```python
from build123d import *

# Parameters (mm, degrees)
SKETCH1_W               = 711.2
SKETCH1_H               = 685.8
BOSS_EXTRUDE1_DEPTH     = 3.175
SKETCH2_W               = 635
SKETCH2_H               = 666.75
BOSS_EXTRUDE2_DEPTH     = 50.8
CUT_EXTRUDE1_DEPTH      = 497.935680571
CUT_EXTRUDE1_DEPTH_BACK = 497.935680571
SKETCH4_W               = 19.05
SKETCH4_H               = 666.75
BOSS_EXTRUDE3_DEPTH     = 3.175
SKETCH5_W               = 317.5
SKETCH5_H               = 6.35
CUT_EXTRUDE2_DEPTH      = 19.05
FILLET1_R               = 43.18
SKETCH6_W               = 635
SKETCH6_H               = 152.4
BOSS_EXTRUDE4_DEPTH     = 15.24
DRAFT2_ANGLE            = 11
SHELL1_START            = -314.325
SHELL1_DEPTH            = 628.65
SHELL1_START_2          = -333.375
SHELL1_2_OUTLINE_W      = 3.175
SHELL1_2_OUTLINE_H      = 663.575
SHELL1_2_DEPTH          = 666.75
SKETCH7_W               = 127
SKETCH7_H               = 127
CUT_EXTRUDE3_DEPTH      = 25.4
LPATTERN1_COUNT         = 4
LPATTERN1_PITCH         = 160.02
FILLET2_R               = 12.7


# Read off the part's stored shape, not the designer's step: Shell1
with BuildPart() as part:
    # Sketch1 → Boss-Extrude1 (new body)
    with BuildSketch(Plane(origin=(0, 0, 0), x_dir=(1, 0, 0), z_dir=(0, 1, 0))):
        Rectangle(SKETCH1_W, SKETCH1_H)
    extrude(amount=BOSS_EXTRUDE1_DEPTH)

    # Sketch2 → Boss-Extrude2 (add)
    with BuildSketch(Plane(origin=(0, 3.175, 0), x_dir=(1, 0, 0), z_dir=(0, 1, 0))):
        with Locations((0, 9.525)):
            Rectangle(SKETCH2_W, SKETCH2_H)
    extrude(amount=BOSS_EXTRUDE2_DEPTH)

    # Sketch3 → Cut-Extrude1 (cut, two sides: drawn at the far end of the back side and taken through both)
    with BuildSketch(Plane(origin=(0, 0, 0), x_dir=(0, 0, -1), z_dir=(1, 0, 0)).offset(-CUT_EXTRUDE1_DEPTH_BACK)):
        Polygon((-196.85, 53.975), (-170.68027758, 44.45), (342.9, 44.45), (342.9, 53.975), align=None)
    extrude(amount=CUT_EXTRUDE1_DEPTH + CUT_EXTRUDE1_DEPTH_BACK, mode=Mode.SUBTRACT)

    # Sketch4 → Boss-Extrude3 (add)
    with BuildSketch(Plane(origin=(0, 3.175, 0), x_dir=(1, 0, 0), z_dir=(0, 1, 0))):
        with Locations((-327.025, 9.525)):
            Rectangle(SKETCH4_W, SKETCH4_H)
    boss_extrude3 = extrude(amount=BOSS_EXTRUDE3_DEPTH)

    # Mirror1: Boss-Extrude3 across plane
    add(boss_extrude3.mirror(Plane(origin=(0, 0, 0), x_dir=(0, 0, 1), z_dir=(1, 0, 0))))

    # Sketch5 → Cut-Extrude2 (cut)
    with BuildSketch(Plane(origin=(0, 0, -342.9), x_dir=(-1, 0, 0), z_dir=(0, 0, -1))):
        with Locations((-158.75, 41.275)):
            Rectangle(SKETCH5_W, SKETCH5_H)
    cut_extrude2 = extrude(amount=-CUT_EXTRUDE2_DEPTH, mode=Mode.SUBTRACT)

    # Mirror2: Cut-Extrude2 across plane
    add(cut_extrude2.mirror(Plane(origin=(0, 0, 0), x_dir=(0, 0, 1), z_dir=(1, 0, 0))), mode=Mode.SUBTRACT)

    # Fillet1
    fillet1_edges = [part.edges().sort_by_distance(p)[0] for p in [
        (0, 53.975, 323.85),
    ]]
    fillet(fillet1_edges, radius=FILLET1_R)

    # Sketch6 → Boss-Extrude4 (add)
    with BuildSketch(Plane(origin=(0, 44.45, 0), x_dir=(1, 0, 0), z_dir=(0, 1, 0))):
        with Locations((0, 222.25)):
            Rectangle(SKETCH6_W, SKETCH6_H)
    extrude(amount=BOSS_EXTRUDE4_DEPTH)

    # Draft2
    draft2_faces = [part.faces().sort_by_distance(p)[0] for p in [
        (0, 52.07, -146.05),
        (0, 52.07, -298.45),
    ]]
    draft(draft2_faces, Plane.ZX.offset(59.69), DRAFT2_ANGLE)

    # Shell1 outline → Shell1 (cut)
    with BuildSketch(Plane.YZ.offset(SHELL1_START)):
        with BuildLine():
            Line((41.275, -145.704912114), (41.275, 171.240115743))
            Line((41.275, 171.240115743), (50.8, 197.409838164))
            Line((50.8, 197.409838164), (50.8, 280.67))
            ThreePointArc((50.8, 280.67), (39.082806781, 308.957806781), (10.795, 320.675))
            Line((10.795, 320.675), (0, 320.675))
            Line((0, 320.675), (0, -342.9))
            Line((0, -342.9), (34.925, -342.9))
            Line((34.925, -342.9), (34.925, -320.675))
            Line((34.925, -320.675), (41.275, -320.675))
            Line((41.275, -320.675), (41.275, -298.795087886))
            Line((41.275, -298.795087886), (56.515, -295.832731975))
            Line((56.515, -295.832731975), (56.515, -148.667268025))
            Line((56.515, -148.667268025), (41.275, -145.704912114))
        make_face()
    extrude(amount=SHELL1_DEPTH, mode=Mode.SUBTRACT)

    # Shell1 2 outline → Shell1 2 (cut)
    with BuildSketch(Plane.YZ.offset(SHELL1_START_2)):
        with Locations((1.5875, -11.1125)):
            Rectangle(SHELL1_2_OUTLINE_W, SHELL1_2_OUTLINE_H)
    extrude(amount=SHELL1_2_DEPTH, mode=Mode.SUBTRACT)

    # Sketch7 → Cut-Extrude3 (cut)
    with BuildSketch(Plane(origin=(0, 59.69, 0), x_dir=(1, 0, 0), z_dir=(0, 1, 0))):
        with Locations((-241.3, 222.25)):
            Rectangle(SKETCH7_W, SKETCH7_H)
    cut_extrude3 = extrude(amount=-CUT_EXTRUDE3_DEPTH, mode=Mode.SUBTRACT)

    # LPattern1: Cut-Extrude3 ×4
    with Locations(*[(i * LPATTERN1_PITCH, 0, 0) for i in range(1, LPATTERN1_COUNT)]):
        add(cut_extrude3, mode=Mode.SUBTRACT)

    # Fillet2
    fillet2_edges = [part.edges().sort_by_distance(p)[0] for p in [
        (-304.8, 58.1025, -158.75),
        (-304.8, 58.1025, -285.75),
        (-177.8, 58.1025, -285.75),
        (-177.8, 58.1025, -158.75),
    ]]
    fillet(fillet2_edges, radius=FILLET2_R)


solid = part.part
```
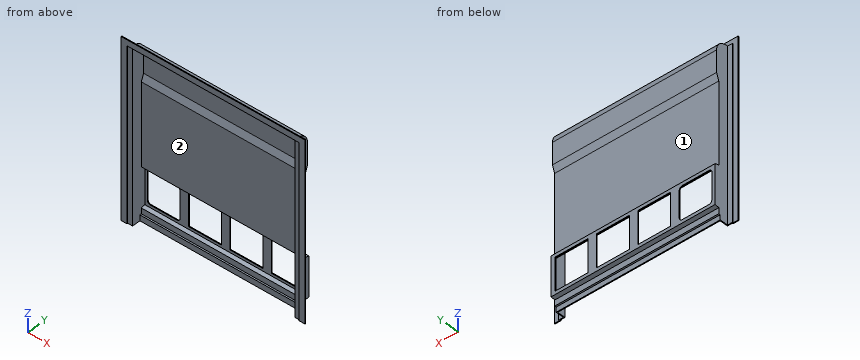
Input: part model. Units: mm. Frame: model coordinates. Face numbers are marked on the shaded views. Give positions to 0.01 mm unless a question says otherwise; leave off trailing zeros. Write each loop counter-clockwise with the first axis right and the second up, starting at its lowest first coordinate (ties: lowest second). Pieces come first, ordered by that corner, then holes. Notation, with made-up numbers: (-19.5, 54.5) - (8.5, 54.5) arc R24 ccw to (8.5, 65.5) - close; hole circle Ø1 at (65.25, 39.5). An arc over 180 degrees is marked (long way). Write item = value, one per line. Start each with the question number.
1) Material intervals for L1, parallel to Z at x = -94, y = 57; L2, parallel to X at y = 40, z = -42.5 (3 decimals); L3, parallel to X at y = 3.5, z = -285 (3 decimals), sorted ascending. Write a range as [from, to].
2) Cut plane B-B (z = 5). Return loops of the section in (x, y) (3 decimals).
3) Draft query along X for the marked faces 1 and 2. Return one class per face: pulls with the +X half, pulls with the -X half, needs draft (parallel to the pull), parting line crosses it, or undercut.
4) Cut plane C-C (x = 156). Return loops of the section in (y, z) (3 decimals), and give its area (3 significant figures).
5) Pin query (flat end, axial travel): pin 1 (4 mm diameter, centred on x = -123, y = 8.5, fed in from +Z); pin 2 (1.6 mm diameter, centred on y = 58, z = -228, fed in from -X); pin 3 (8 mm diameter, centred on y = 18.5, z = 196, fed in from +X). Return the tip coordinate at first contact, or that it passes through.
6) Cut plane D-D (y = 20.5). Return loops of the section in (x, z) (3 decimals).
Answers follow:
q1.L1 = [-298.97, -285.75], [-158.75, -145.53]
q1.L2 = [-317.5, -314.325], [314.325, 317.5]
q1.L3 = [-336.55, -314.325], [314.325, 336.55]
q2.outline = (-355.6, 0) - (-333.375, 0) - (-333.375, 3.175) - (-314.325, 3.175) - (-314.325, 41.275) - (314.325, 41.275) - (314.325, 3.175) - (333.375, 3.175) - (333.375, 0) - (355.6, 0) - (355.6, 3.175) - (336.55, 3.175) - (336.55, 6.35) - (317.5, 6.35) - (317.5, 44.45) - (-317.5, 44.45) - (-317.5, 6.35) - (-336.55, 6.35) - (-336.55, 3.175) - (-355.6, 3.175) - close
q3.face_1 = needs draft
q3.face_2 = undercut
q4.outline = (0, 320.675) - (10.795, 320.675) arc R40.005 cw to (50.8, 280.67) - (50.8, 197.41) - (41.275, 171.24) - (41.275, -145.705) - (56.515, -148.667) - (56.515, -295.833) - (41.275, -298.795) - (41.275, -320.675) - (34.925, -320.675) - (34.925, -342.9) - (38.1, -342.9) - (38.1, -323.85) - (44.45, -323.85) - (44.45, -301.412) - (59.69, -298.45) - (59.69, -146.05) - (44.45, -143.088) - (44.45, 170.68) - (53.975, 196.85) - (53.975, 280.67) arc R43.18 ccw to (10.795, 323.85) - (3.175, 323.85) - (3.175, 342.9) - (0, 342.9) - close
q4.area = 2,390 mm^2
q5.pin_1 = 323.85
q5.pin_2 = -317.5
q5.pin_3 = 317.5
q6.outline = (-317.5, -342.9) - (-314.325, -342.9) - (-314.325, 319.48) - (314.325, 319.48) - (314.325, -342.9) - (317.5, -342.9) - (317.5, 322.745) - (-317.5, 322.745) - close
